Geometry: see drawing. Coordinates: mm, zero at the bounding-box minimum. A direction names the side the tool comes from. Round coordinates to 2 decimals unless told otherwise and drop trailing zeros. Write each loop counter-clockwise with the first axis right and the second up, starting at its lowest first coordinate (ties: lowest second). Pieces come first, ordered by that corner, then holes. Notation, with made-up numbers: (53, 8.25) - (82, 8.25) arc R25 cw to (82, 29.25) - close; hole circle Ø8 at (4, 4). An arc over 180 degrees is marked (long way). One line per item, written item: value. Start each with the question number.
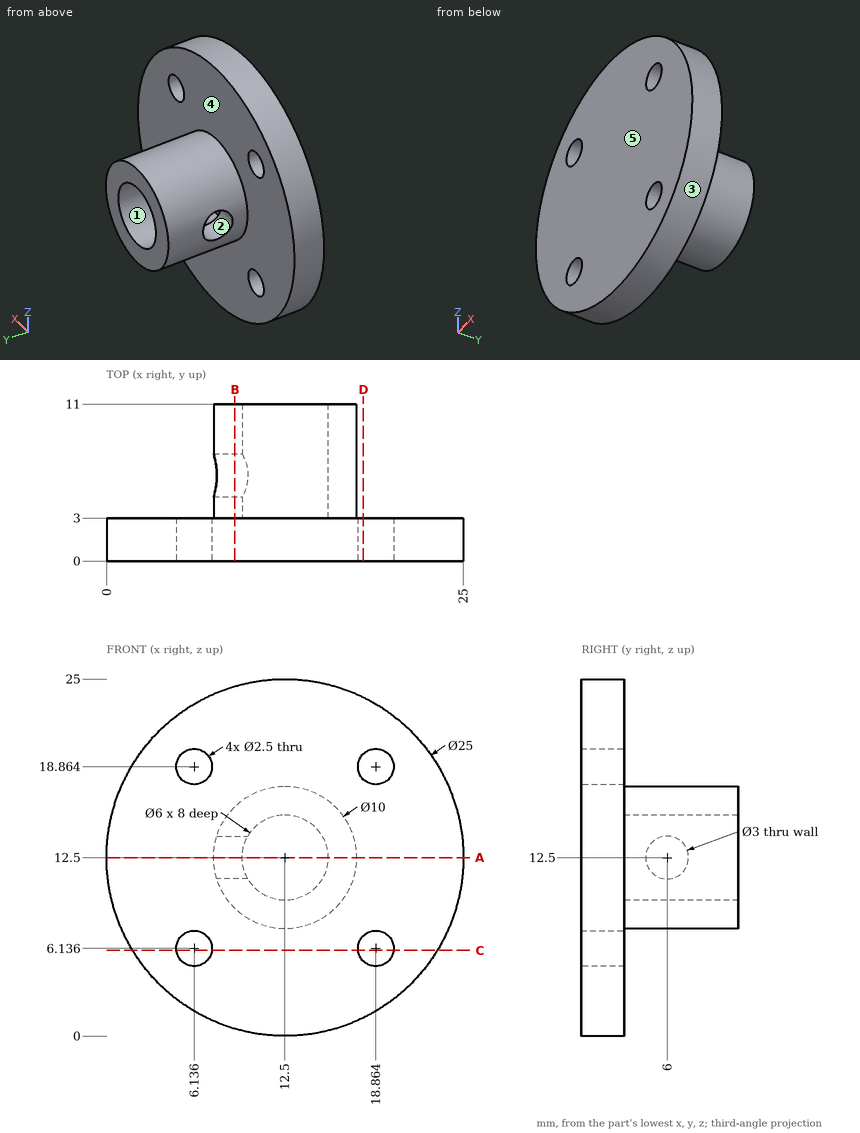
Q1. Cut plane D-D, the plane x = 18. Output: boundary loops of the cut face in (y, z) (3 decimals), and give its area (3 significant figures).
Q2. Material intervals for probe 1 along X at (y, z) = (8.5, 12.5); probe 2 along Z at (x, y) = (19.25, 1.75) (3 decimals); probe 3 along Y at (x, z) = (3, 5.25), sorted ascending. Write a range as from..to.
Q3. Cut plane B-B, the plane x = 9. Output: boundary loops of the cut face in (y, z).
Q4. Access query for the marked faces 4 and 5. Directions: +Z, -Z, +X, -X, +Y, -Y. A direction counts if a zero-diameter tool reaches every point of the face in a straight line with its end or side. Return the directions, or none.
Q5. Contact query for flat-ended pins moving along their axis: pin 1 Ø1 at (y, z) = (6.5, 11.5) entering from +X (3 decimals); pin 2 Ø3 at (x, z) = (10.5, 11.5) entering from +Y; pin 3 Ø3 at (x, z) = (6.14, 6.14) entering from +Y; pin 4 Ø1.8 at (y, z) = (6, 12.5) entering from -X. Output: stop coordinate, or through.
Q6. Cut plane C-C, the plane z = 6. Output: boundary loops of the cut face in (x, y).
Q7. Pull-direction query (X, two-part tool) for the marked faces 1, 2 and 3; classes: pulls with the +X half, pulls with the -X half, needs draft (parallel to the pull), parting line crosses it, or undercut.
Q8. Cut plane A-A, the plane z = 12.5. Output: boundary loops of the cut face in (x, y), and give its area (3 significant figures).
A:
1. outline: (0, 1.275) - (3, 1.275) - (3, 5.233) - (0, 5.233) - close; (0, 7.039) - (3, 7.039) - (3, 17.961) - (0, 17.961) - close; (0, 19.767) - (3, 19.767) - (3, 23.725) - (0, 23.725) - close
1. area: 56.5 mm²
2. probe 1: x = 7.5..9.5, 15.5..17.5
2. probe 2: z = 1.979..4.947, 7.325..17.675, 20.053..23.021
2. probe 3: y = 0..3
3. outline: (0, 0.5) - (3, 0.5) - (3, 8.93) - (11, 8.93) - (11, 16.07) - (3, 16.07) - (3, 24.5) - (0, 24.5) - close; hole circle Ø3 at (6, 12.5)
4. face 4: +Y
4. face 5: +Z, -Z, +X, -X, -Y
5. pin 1: stops at x = 17.475
5. pin 2: stops at y = 11
5. pin 3: stops at y = 3
5. pin 4: stops at x = 15.36
6. outline: (1.82, 0) - (4.89, 0) - (4.89, 3) - (1.82, 3) - close; (7.38, 0) - (17.62, 0) - (17.62, 3) - (7.38, 3) - close; (20.11, 0) - (23.18, 0) - (23.18, 3) - (20.11, 3) - close
7. face 1: undercut
7. face 2: needs draft
7. face 3: parting line crosses it
8. outline: (0, 0) - (25, 0) - (25, 3) - (17.5, 3) - (17.5, 11) - (15.5, 11) - (15.5, 3) - (9.5, 3) - (9.5, 4.5) - (7.5, 4.5) - (7.5, 3) - (0, 3) - close; (7.5, 7.5) - (9.5, 7.5) - (9.5, 11) - (7.5, 11) - close
8. area: 101 mm²
